Verification items for the finished model (mm, model axes). Coordinates: 2 decimals unless noted, no trailing zeros. Write each loop counter-clockwise with the first axis right and the second up, starting at its lowest first coordinate (ties: lowest second). Pieces come first, ordered by that corner, then holes.
```python
from build123d import *

# Parameters (mm, degrees)
F1_DEPTH = 3
F2_R     = 2.375
F3_DEPTH = 2.5


with BuildPart() as f1:
    # F0 (on Top) → F1 (new body)
    with BuildSketch(Plane.XY):
        with BuildLine():
            ThreePointArc((16.625, -9.309773), (32.75, 0), (16.625, 9.309773))
            ThreePointArc((16.625, 9.309773), (5.375, 9.309773), (-0.25, 19.052559))
            ThreePointArc((-0.25, 19.052559), (-16.375, 28.362332), (-16.375, 9.742786))
            ThreePointArc((-16.375, 9.742786), (-10.75, 0), (-16.375, -9.742786))
            ThreePointArc((-16.375, -9.742786), (-16.375, -28.362332), (-0.25, -19.052559))
            ThreePointArc((-0.25, -19.052559), (5.375, -9.309773), (16.625, -9.309773))
        make_face()
    extrude(amount=F1_DEPTH)

    # F2 (on face) → F3 (join)
    with BuildSketch(Plane.XY.offset(3)):
        Circle(F2_R)
    extrude(amount=F3_DEPTH)


solid = f1.part
```
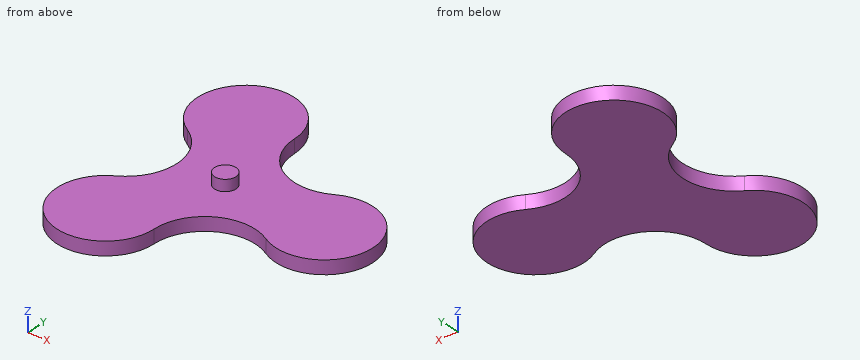
1. Sectioned sample at D-D, the plane x = 22. Record the boundary of the cut face in (y, z).
2. Gauge pin test, flat ends, axial feed: P1, Ø2, axis at x = -8, y = -11.5, coming from the +Z side; P2, Ø2, axis at y = 15, z = 3, coming from the +X side. Record the tip position at first contact, or that the pin passes through.
3. Sectioned sample at B-B, the plane x = -12. Record the boundary of the cut face in (y, z).
4. Sectioned sample at C-C, the plane z = 1.9. Record the boundary of the cut face in (x, y) (3 decimals).
5. Material ranges on L1, parallel to Z at x = -4.5, y = 11.5; L2, parallel to Y at x = -12, z = 1; L3, parallel to Y at x = -15.5, z = 0.85, recorded low to high.
6. Sectioned sample at A-A, the plane y = 0. Record the boundary of the cut face in (x, z) (3 decimals), and give its area (3 significant figures).
Outcome:
1. outline: (-10.75, 0) - (10.75, 0) - (10.75, 3) - (-10.75, 3) - close
2. P1: stops at z = 3
2. P2: stops at x = 0.95
3. outline: (-29.76, 0) - (-5.15, 0) - (-5.15, 3) - (-29.76, 3) - close; (5.15, 0) - (29.76, 0) - (29.76, 3) - (5.15, 3) - close
4. outline: (-16.375, -9.743) arc R10.75 ccw (long way) to (-0.25, -19.053) arc R11.25 cw to (16.625, -9.31) arc R10.75 ccw (long way) to (16.625, 9.31) arc R11.25 cw to (-0.25, 19.053) arc R10.75 ccw (long way) to (-16.375, 9.743) arc R11.25 cw to start
5. L1: z = 0 to 3
5. L2: y = -29.76 to -5.15, 5.15 to 29.76
5. L3: y = -28.82 to -9.18, 9.18 to 28.82
6. outline: (-10.75, 0) - (32.75, 0) - (32.75, 3) - (2.375, 3) - (2.375, 5.5) - (-2.375, 5.5) - (-2.375, 3) - (-10.75, 3) - close
6. area: 142 mm2
